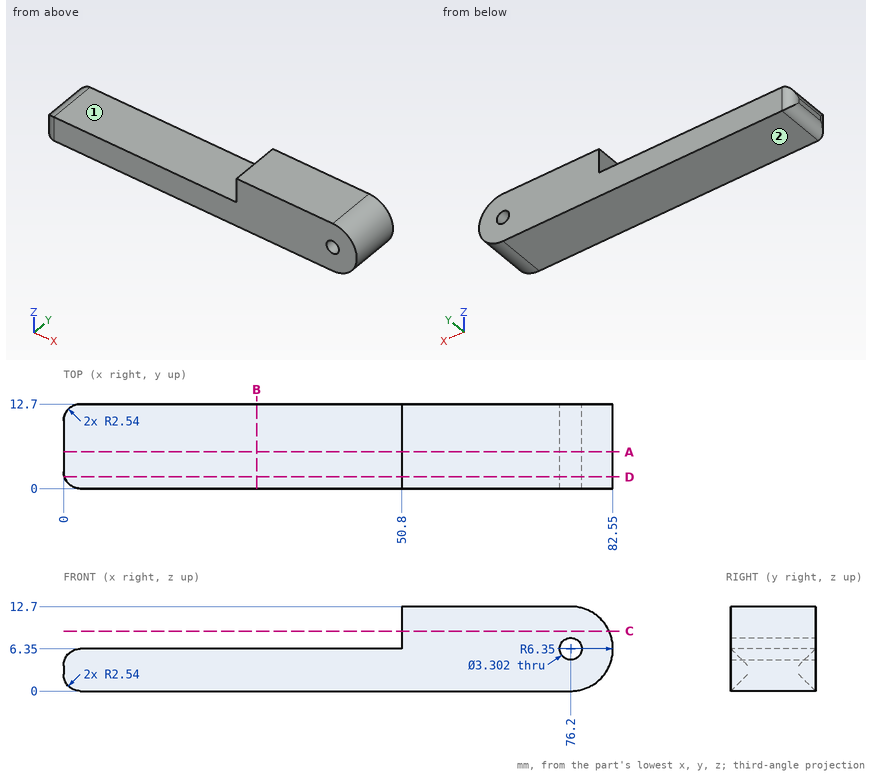
Drawing for the job (mm, zero at the part's lowest x, y, z). A direction names the side the tool comes from. Give positions to 0.01 mm unless a question says otherwise; leave off trailing zeros. Write each loop counter-clockwise with the first axis right and the second up, starting at its lowest first coordinate (ties: lowest second). Pieces come first, ordered by that corner, then holes. Notation, with made-up numbers: M 80,0.25 L 95,0.25 A22 ccw 95,33.25 Z; hole C 9,-1 d9. An arc over 180 degrees is marked long. Return JSON: item names as keys, results as strings. Group by question number.
(1) Band-saw the part on C-C (z = 9). Give the cut face in (x, y).
(2) Flat gauge pins, fed straight in: pin 1 Ø4 at (x, y) = (20, 5) entering from +Z; pin 2 Ø1.9 at (y, z) = (3.5, 10) entering from -X. Where does each tip first touch, or does it go through?
(3) Band-saw the part on B-B (x = 29). Give the cut face in (y, z).
(4) Drill centre lines: L1, parallel to Z at x = 76.2, y = 4.5; L2, parallel to Z at x = 22.5, y = 6.5; L3, parallel to X at y = 9.5, z = 7.5 (3 decimals). Where is each one in solid material? Low to high. Write a range as [from, to].
(5) Band-saw the part on D-D (y = 1.75). Give the cut face in (x, z).
(6) Band-saw the part on A-A (y = 5.5). Give the cut face in (x, z), and give its area (3 significant figures).
(7) 3-axis set-ups, long thin cutter, end or side, ignore diameter. For the marked faces 1 and 2: which of +Z, -Z, +X, -X, +Y, -Y reach the whole face in a straight line?
Entries:
{
 "1": {"outline": "M 50.8,0 L 81.97,0 L 81.97,12.7 L 50.8,12.7 Z"},
 "2": {"pin 1": "stops at z = 6.35", "pin 2": "stops at x = 50.8"},
 "3": {"outline": "M 0,0 L 12.7,0 L 12.7,6.35 L 0,6.35 Z"},
 "4": {"L1": "z = [0, 4.7], [8, 12.7]", "L2": "z = [0, 6.35]", "L3": "x = [50.8, 75.015], [77.385, 82.445]"},
 "5": {"outline": "M 0.13,1.75 A2.54 ccw 2.54,0 L 76.2,0 A6.35 ccw 76.2,12.7 L 50.8,12.7 L 50.8,6.35 L 2.54,6.35 A2.54 ccw 0.13,4.6 Z; hole C 76.2,6.35 d3.3"},
 "6": {"outline": "M 0,2.54 A2.54 ccw 2.54,0 L 76.2,0 A6.35 ccw 76.2,12.7 L 50.8,12.7 L 50.8,6.35 L 2.54,6.35 A2.54 ccw 0,3.81 Z; hole C 76.2,6.35 d3.3", "area": "697 mm^2"},
 "7": {"face 1": "+Z, -X, +Y, -Y", "face 2": "-Z, +X, -X, +Y, -Y"}
}
